Autodesk Inventor part; units mm, degrees
ref_plane "YZ Plane" through (0, 0, 0) normal (1, 0, 0) x (0, 1, 0)
ref_plane "XZ Plane" through (0, 0, 0) normal (0, 1, 0) x (-1, 0, 0)
ref_plane "XY Plane" through (0, 0, 0) normal (0, 0, 1) x (1, 0, 0)
sketch "Sketch1" plane through (0, 0, 0) normal (0, 1, 0) x (-1, 0, 0)
  line L0 (0, -234.315) -> (0, 339.09)
  line L1 (-213.36, 0) -> (213.36, 0)
  line L2 (213.36, 0) -> (-213.36, 0)
  line L3 (0, -234.315) -> (0, 339.09)
  line L4 (152.4, 254) -> (-152.4, 254)
  line L5 (-152.4, 254) -> (-152.4, 0)
  line L6 (152.4, 0) -> (152.4, 254)
  arc A0 (-152.4, 0) -> (152.4, 0) centre (0, 0) ccw
  line L7 (111.125, 254) -> (41.275, 254) construction
  line L8 (111.125, 257.175) -> (41.275, 257.175)
  line L9 (41.275, 250.825) -> (111.125, 250.825)
  arc A1 (111.125, 250.825) -> (111.125, 257.175) centre (111.125, 254) ccw
  arc A2 (41.275, 257.175) -> (41.275, 250.825) centre (41.275, 254) ccw
  line L10 (-41.275, 254) -> (-111.125, 254) construction
  line L11 (-41.275, 257.175) -> (-111.125, 257.175)
  line L12 (-111.125, 250.825) -> (-41.275, 250.825)
  arc A3 (-41.275, 250.825) -> (-41.275, 257.175) centre (-41.275, 254) ccw
  arc A4 (-111.125, 257.175) -> (-111.125, 250.825) centre (-111.125, 254) ccw
  circle A5 centre (0, 0) radius 14.2875
  point P0 (76.2, 254)
  point P1 (-76.2, 254)
  point P2 (0, -152.4)
  point P3 (114.3, 254)
  point P4 (38.1, 254)
  dimension "d2" = 69.85
  dimension "d3" = 6.35
  dimension "d4" = 69.85
  dimension "d5" = 6.35
  dimension "d7" = 76.2
  dimension "d8" = 304.8
  dimension "d9" = 76.2
  dimension "d10" = 28.575
  dimension "d11" = 406.4
  dimension "d15" = 76.2
extrude "Extrusion1" add sketch "Sketch1" along normal blind 6.35 contours A0 L1 A5 L0 | L0 A5 L1 A0 | L5 L4 A4 L12 A3 L0 A5 L1 | L1 A5 L0 L4 A2 L9 A1 L6 | A4 L11 A3 L4 | L4 A3 L12 A4 | A1 L9 A2 L4 | L4 A2 L8 A1
sketch "Sketch2" plane through (0, 6.35, 0) normal (0, 1, 0) x (1, 0, 0)
  circle A0 centre (0, 0) radius 57.5
  circle A1 centre (0, -100.33) radius 37.5
  line L0 (-9.8425, -130.5684) -> (9.8425, -130.5684)
  line L1 (9.8425, -130.5684) -> (9.8425, -90.0684)
  line L2 (9.8425, -90.0684) -> (-9.8425, -90.0684)
  line L3 (-9.8425, -90.0684) -> (-9.8425, -130.5684)
  line L4 (0, 234.315) -> (0, -339.09)
  dimension "d16" = 115
  dimension "d17" = 75
  dimension "d18" = 19.685
  dimension "d19" = 40.5
  dimension "d20" = 10.2616
  dimension "d21" = 9.8425
  dimension "d24" = 100.33
extrude "Extrusion2" cut sketch "Sketch2" against normal blind 25.4 contours L4 L0 L3 L2 | L2 L1 L0 L4
sketch "Sketch3" plane through (0, 6.35, 0) normal (0, 1, 0) x (1, 0, 0)
  line L0 (9.8425, -90.0684) -> (9.8425, -130.5684)
  line L1 (9.8425, -130.5684) -> (-9.8425, -130.5684)
  line L2 (-9.8425, -130.5684) -> (-9.8425, -90.0684)
  line L3 (-9.8425, -90.0684) -> (9.8425, -90.0684)
  circle A0 centre (0, 0) radius 14.2875
  line L4 (-38.1, -254) -> (38.1, -254)
  arc A1 (38.1, -254) -> (41.275, -257.175) centre (41.275, -254) ccw
  line L5 (41.275, -257.175) -> (111.125, -257.175)
  arc A2 (111.125, -257.175) -> (114.3, -254) centre (111.125, -254) ccw
  line L6 (114.3, -254) -> (152.4, -254)
  line L7 (152.4, -254) -> (152.4, 0)
  arc A3 (152.4, 0) -> (-152.4, 0) centre (0, 0) ccw
  line L8 (-152.4, 0) -> (-152.4, -254)
  line L9 (-152.4, -254) -> (-114.3, -254)
  arc A4 (-114.3, -254) -> (-111.125, -257.175) centre (-111.125, -254) ccw
  line L10 (-111.125, -257.175) -> (-41.275, -257.175)
  arc A5 (-41.275, -257.175) -> (-38.1, -254) centre (-41.275, -254) ccw
  line L11 (152.4, -177.8) -> (152.4, 0)
  line L12 (14.2875, 0) -> (-14.2875, 0)
  line L13 (-152.4, 0) -> (-152.4, -177.8)
  arc A6 (152.4, 0) -> (-152.4, 0) centre (0, 0) ccw
  line L14 (-152.4, -177.8) -> (-152.4, 0) construction
  line L15 (-152.4, 0) -> (0, 152.4) construction
  line L16 (0, 152.4) -> (152.4, 0) construction
  line L17 (152.4, 0) -> (152.4, -177.8) construction
  spline S0 degree 4 poles (-152.4, -177.8) (-152.4, 0) (0, 152.4) (152.4, 0) (152.4, -177.8) knots 1 1 1 1 1 2 2 2 2 2
  line L18 (152.4, -177.8) -> (152.4, 0)
  line L19 (-152.4, 0) -> (-152.4, -177.8)
extrude "Extrusion3" cut sketch "Sketch3" against normal blind 25.4 contours L8 A3 L7 S0
properties part number "turretSidePlateOne"
The model under review builds one solid part; all positions refer to its coordinate system, in mm. A direction names the side the tool comes from. Round coordinates to 2 decimals unless told otherwise and drop trailing zeros. Answer as a JSON object with one key per item and string values.
1. We need section A-A on y = 3.5. State how many separate pieces and enclosed holes the cut face has, and give its area (3 significant figures).
Results found:
{"separate pieces": "1", "enclosed holes": "2", "area": "72,900 mm^2"}
2. To check wall thickness, follow line 1 along X through (y, z) = (4.5, 0); line 2 along X through (y, z) = (4.75, 122); line 3 along Z through (x, y) = (-118, 2.25). State the ranges of each line that lie inside material, in increasing order.
Results found:
{"line 1": "x = -82.57 to -14.29, 14.29 to 82.57", "line 2": "x = -146.77 to -9.84, 9.84 to 146.77", "line 3": "z = 44.91 to 254"}
3. The part is to be moulded in two halves that separate along X. For faces 4 (the face through (14.274, 3.131, -0.628)), 5 (the face through (152.4, 3, 216)), 6 (the face through (-77, 3, 257.175)), say which applies: pulls with the +X half, pulls with the -X half, needs draft (parallel to the pull), parting line crosses it, or undercut.
Results found:
{"face 4": "undercut", "face 5": "pulls with the +X half", "face 6": "needs draft"}
4. Machinability: for faces 1 (the face through (-134, 3, 254)), 2 (the face through (0, 3, 90.068)), 3 (the face through (133, 3, 254)), which of the approach directions +Z, -Z, +X, -X, +Y, -Y give a long, thin tool a straight path to every point of the face, cutting with its end or side? Answer none if there is none.
Results found:
{"face 1": "+Z, -X, +Y, -Y", "face 2": "+Y, -Y", "face 3": "+Z, +X, +Y, -Y"}
5. Clearance check with flat-ended pins moving along their axes: pin 1 (10 mm diameter, centred on x = -51, z = 205.5, fed in from -Y); pin 2 (1.9 mm diameter, centred on y = 4, z = 108.5, fed in from +X); pin 3 (1.5 mm diameter, centred on x = -3, y = 3, fed in from +Z). State where each tip first meets the part, or that it passes through.
Results found:
{"pin 1": "stops at y = 0", "pin 2": "stops at x = 143.91", "pin 3": "stops at z = 254"}
